The listing builds one solid part. Answer for the finished solid, in the listing's coordinates (mm). A direction names the side the tool comes from. Give positions to 0.01 mm unless a question says otherwise; leave off trailing zeros. Write each loop counter-clockwise with the first axis right and the second up, starting at its lowest first coordinate (ties: lowest second). Pieces come first, ordered by that corner, then holes. Notation, with made-up numbers: (33, 79) -> (45, 79) arc R20 cw to (45, 99) -> close; hole circle Ø8 at (-15.5, 27). An arc over 180 degrees is marked (long way). Write each question's results on one line, items separated by ' | '. Start each with the question number.
from build123d import *

# Parameters (mm, degrees)
F1_DEPTH = 25.4
F3_DEPTH = 12.7
F5_DEPTH = 25.4
F7_DEPTH = 25.4
F9_DEPTH = 12.7


with BuildPart() as f1:
    # F0 (on Front) → F1 (new body)
    with BuildSketch(Plane.XZ):
        Polygon((-37.9636640911, -15.4334478322), (-50.6636640911, -15.4334478322), (-50.6636640911, -28.1334478322), (0.1363359089, -28.1334478322), (0.1363359089, -15.4334478322), (-12.5636640911, -15.4334478322), (-12.5636640911, 3.6165521678), (-37.9636640911, 3.6165521678), align=None)
    extrude(amount=F1_DEPTH)

    # F2 (on face) → F3 (join)
    with BuildSketch(Plane.XY.offset(-15.4334478322)):
        with BuildLine():
            ThreePointArc((12.8363359089, -12.7), (9.11659203, -3.7197438789), (0.1363359089, 0))
            Line((0.1363359089, 0), (0.1363359089, -12.7))
            Line((0.1363359089, -12.7), (12.8363359089, -12.7))
        make_face()
        with BuildLine():
            Line((12.8363359089, -12.7), (0.1363359089, -12.7))
            Line((0.1363359089, -12.7), (0.1363359089, -25.4))
            ThreePointArc((0.1363359089, -25.4), (9.11659203, -21.6802561211), (12.8363359089, -12.7))
        make_face()
        with BuildLine():
            Line((-50.6636640911, -12.7), (-50.6636640911, 0))
            ThreePointArc((-50.6636640911, 0), (-59.6439202122, -3.7197438789), (-63.3636640911, -12.7))
            Line((-63.3636640911, -12.7), (-50.6636640911, -12.7))
        make_face()
        with BuildLine():
            Line((-50.6636640911, -25.4), (-50.6636640911, -12.7))
            Line((-50.6636640911, -12.7), (-63.3636640911, -12.7))
            ThreePointArc((-63.3636640911, -12.7), (-59.6439202122, -21.6802561211), (-50.6636640911, -25.4))
        make_face()
    extrude(amount=-F3_DEPTH)

    # F4 (on face) → F5 (join)
    with BuildSketch(Plane.YZ.offset(-12.5636640911)):
        with BuildLine():
            ThreePointArc((-12.7, 16.3165521678), (-21.6802561211, 12.5968082888), (-25.4, 3.6165521678))
            Line((-25.4, 3.6165521678), (-12.7, 3.6165521678))
            Line((-12.7, 3.6165521678), (-12.7, 16.3165521678))
        make_face()
        with BuildLine():
            Line((-12.7, 16.3165521678), (-12.7, 3.6165521678))
            Line((-12.7, 3.6165521678), (0, 3.6165521678))
            ThreePointArc((0, 3.6165521678), (-3.7197438789, 12.5968082888), (-12.7, 16.3165521678))
        make_face()
    extrude(amount=-F5_DEPTH)

    # F6 (on face) → F7 (cut)
    with BuildSketch(Plane.YZ.offset(-12.5636640911)):
        with BuildLine():
            ThreePointArc((-6.35, 3.6165521678), (-8.2098719395, 8.1066802283), (-12.7, 9.9665521678))
            ThreePointArc((-12.7, 9.9665521678), (-17.1901280605, 8.1066802283), (-19.05, 3.6165521678))
            ThreePointArc((-19.05, 3.6165521678), (-12.7, -2.7334478322), (-6.35, 3.6165521678))
        make_face()
    extrude(amount=-F7_DEPTH, mode=Mode.SUBTRACT)

    # F8 (on face) → F9 (cut)
    with BuildSketch(Plane.XY.offset(-15.4334478322)):
        with BuildLine():
            ThreePointArc((-44.3136640911, -12.7), (-46.1735360306, -8.2098719395), (-50.6636640911, -6.35))
            ThreePointArc((-50.6636640911, -6.35), (-55.1537921516, -8.2098719395), (-57.0136640911, -12.7))
            ThreePointArc((-57.0136640911, -12.7), (-55.1537921516, -17.1901280605), (-50.6636640911, -19.05))
            ThreePointArc((-50.6636640911, -19.05), (-46.1735360306, -17.1901280605), (-44.3136640911, -12.7))
        make_face()
        with BuildLine():
            ThreePointArc((0.1363359089, -19.05), (4.6264639694, -17.1901280605), (6.4863359089, -12.7))
            ThreePointArc((6.4863359089, -12.7), (4.6264639694, -8.2098719395), (0.1363359089, -6.35))
            ThreePointArc((0.1363359089, -6.35), (-6.2136640911, -12.7), (0.1363359089, -19.05))
        make_face()
    extrude(amount=-F9_DEPTH, mode=Mode.SUBTRACT)


solid = f1.part
1. Consider probe 1 along X at (y, z) = (-13.75, -21.5); probe 2 along X at (y, z) = (-9, -3.5); probe 3 along Y at (x, z) = (-24, 1). Determine where each line is inside the solid, lowest interval first. Write a range as [from, to].
2. Section A-A (x = -16) is taken. Write down the section's boundary in (y, z).
3. The mould has two halves that part along Y. Classify faces 4 (the flat face through (-26, -25.4, -16)), 5 (the flat face through (-37.964, -13, -3)), 6 (the flat face through (-26, 0, -16)): pulls with the +Y half, pulls with the -Y half, needs draft (parallel to the pull), parting line crosses it, or undercut.
4. Section C-C (z = -20) is taken. Write down the section's boundary in (x, y).
5. A tool of negligible diameter and unlimited length cuts with its end or side. For faces 1 (the flat face through (-44.8, -9.7, -15.433)), 2 (the flat face through (-6, -15, -15.433)), 3 (the flat face through (-26, -13, -28.133)), from which of +Z, -Z, +X, -X, +Y, -Y can it reach the whole face along a straight path? Write none if from no direction.
6. Each of these flat-tipped pins is pushed along its axis until it touches: pin 1 Ø8 at (y, z) = (-22, -13.5) entering from -X; pin 2 Ø3 at (x, y) = (-3.5, -19.5) entering from +Z; pin 3 Ø2 at (y, z) = (-16.5, -7) entering from -X. Where does it stop, or does it pass through?
7. Section D-D (x = -46) is taken. Write down the section's boundary in (y, z).
8. Section B-B (y = -16.75) is taken. Write down the section's boundary in (x, z).
Results:
1) probe 1: x = [-63.32, -56.93], [-44.4, -6.13], [6.4, 12.79] | probe 2: x = [-37.96, -12.56] | probe 3: y = [-25.4, -18.49], [-6.91, 0]
2) outline: (-25.4, -28.13) -> (0, -28.13) -> (0, 3.62) arc R12.7 ccw to (-25.4, 3.62) -> close; hole circle Ø12.7 at (-12.7, 3.62)
3) face 4: pulls with the -Y half | face 5: needs draft | face 6: pulls with the +Y half
4) outline: (-50.66, -25.4) -> (0.14, -25.4) arc R12.7 ccw to (0.14, 0) -> (-50.66, 0) arc R12.7 ccw to start; hole circle Ø12.7 at (-50.66, -12.7); hole circle Ø12.7 at (0.14, -12.7)
5) face 1: +Z, -X, +Y, -Y | face 2: +Z, +X, +Y, -Y | face 3: -Z, +X, -X, +Y, -Y
6) pin 1: stops at x = -61.96 | pin 2: stops at z = -15.43 | pin 3: stops at x = -37.96
7) outline: (-25.4, -28.13) -> (-17.01, -28.13) -> (-17.01, -15.43) -> (-25.4, -15.43) -> close; (-8.39, -28.13) -> (0, -28.13) -> (0, -15.43) -> (-8.39, -15.43) -> close
8) outline: (-62.7, -28.13) -> (-55.55, -28.13) -> (-55.55, -15.43) -> (-62.7, -15.43) -> close; (-45.77, -28.13) -> (-4.75, -28.13) -> (-4.75, -15.43) -> (-12.56, -15.43) -> (-12.56, -1.27) -> (-37.96, -1.27) -> (-37.96, -15.43) -> (-45.77, -15.43) -> close; (-37.96, 8.51) -> (-12.56, 8.51) -> (-12.56, 15.65) -> (-37.96, 15.65) -> close; (5.03, -28.13) -> (12.17, -28.13) -> (12.17, -15.43) -> (5.03, -15.43) -> close
